from build123d import *

# Parameters (mm, degrees)
F1_DEPTH    = 3.175
F5_DEPTH    = 3.175
F6_T1_DEPTH = 117.475


# Not quite as in the source:
# - a fillet or chamfer that OpenCascade refuses, or shapes differently, is made with other operations: its cross-section is extruded or revolved along the edge and cut away or added


with BuildPart() as f1:
    # F0 (on Top) → F1 (new body)
    with BuildSketch(Plane.XY):
        Polygon((50.8, 0), (0, 87.9881810245), (-50.8, 0), align=None)
    extrude(amount=F1_DEPTH)

    # F4 (on line) → F5 (join)
    with BuildSketch(Plane(origin=(30.2473107364, 17.7959839325, 17.4632910558), x_dir=(-0.3931673168, 0.8910065242, -0.226995231), z_dir=(0.7716343063, 0.4539904997, 0.445503225))):
        Polygon((6.5029600393, 75.2459340132), (-19.9755570322, -25.4006840255), (78.3980433443, 0), align=None)
    extrude(amount=F5_DEPTH)

    # F6: fillet of radius 3.175 on 1 edges, made by hand

    # F6_s2 → F6_t1 (cut)
    with BuildSketch(Plane(origin=(17.005719551, -29.012184774, 0.1101218851), x_dir=(-0.862716434, -0.5056880012, 0), z_dir=(-0.5056852899, 0.8627118085, -0.0032746052))):
        with BuildLine():
            ThreePointArc((-45.25402581, 4.1728704395), (-45.421662158, 1.7486197382), (-43.8259948462, -0.0841211704))
            Line((-43.8259948462, -0.0841211704), (-46.668506133, 1.3303591527))
            Line((-46.668506133, 1.3303591527), (-45.25402581, 4.1728704395))
        make_face()
    extrude(amount=F6_T1_DEPTH, mode=Mode.SUBTRACT)


solid = f1.part
Verification items for the finished model (mm, model axes). A direction names the side the tool comes from. Coordinates: 2 decimals unless noted, no trailing zeros. Loops run counter-clockwise (first coordinate to the right, second up) from the corner with the lowest first, then second, coordinate; pieces in that order, holes last. Notation, with made-up numbers: (60.5, -36.75) -> (101.5, -36.75) arc R22 cw to (101.5, -3.75) -> close; hole circle Ø3 at (60, -35.5). An arc over 180 degrees is marked (long way). Write each question's results on one line, items separated by ' | '.
Item 1: Section check C-C, the plane x = -43. Enter the section's corners in (y, z) (3 decimals).
Found:
outline: (0, 0) -> (13.51, 0) -> (13.51, 3.175) -> (0, 3.175) -> close
Item 2: Material ranges on L1, parallel to Z at x = -9.5, y = 49 (3 decimals); L2, parallel to Z at x = 1, y = 75.5 (3 decimals); L3, parallel to Z at x = 17.5, y = 13 (3 decimals), recorded low to high.
Found:
L1: z = 0 to 3.175 | L2: z = 0 to 3.175, 9.318 to 16.445 | L3: z = 0 to 3.175, 44.43 to 44.627
Item 3: Section check B-B, the plane z = 55. Enter the section's corners in (x, y).
Found:
outline: (-6.93, 44.15) -> (9.64, 15.99) -> (13.15, 17.02) -> (-4.32, 46.7) -> close
Item 4: Gauge pin test, flat ends, axial feed: pin 1 (5 mm diameter, centred on y = 72, z = 17.5, fed in from +X); pin 2 (2 mm diameter, centred on x = 33, z = 14, fed in from -Y); pin 3 (1.5 mm diameter, centred on y = 16.5, z = 15, fed in from -X). Record the tip position at first contact, or that the pin passes through.
Found:
pin 1: stops at x = 4.51 | pin 2: stops at y = 14.55 | pin 3: stops at x = 31.81
Item 5: Mould release check, pull along Z, two halves, no side actions. Record for faces 1 (the face through (21.22, 12.67, 41.84)), 2 (the face through (-1, 35, 3.175)), 3 (the face through (-1, 0, 2)): +Z half, -Z half, draft (parallel to the pull), parting line (faces both ways), or undercut.
Found:
face 1: +Z half | face 2: undercut | face 3: draft
Item 6: Tool access check on faces 4 (the face through (17.65, 34.57, 29.32)), 5 (the face through (15.13, 32.99, 28.16)), 6 (the face through (-1, 35, 0)). Record the directions out of +Z, -Z, +X, -X, +Y, -Y that give a thin tool (end or side, any length) a straight path to the whole face; none if there is none.
Found:
face 4: +Z, +X, +Y | face 5: -X, -Y | face 6: -Z, -X, -Y
Item 7: Section check A-A, the plane x = -5. Enter the section's corners in (y, z) (3 decimals), plus the area to 3 significant figures.
Found:
outline: (0, 0) -> (79.328, 0) -> (79.328, 3.175) -> (0, 3.175) -> close; (21.674, 74.561) -> (57.361, 38.195) -> (42.028, 60.946) -> (24.067, 79.249) -> close | area: 443 mm2
